from build123d import *

# Parameters (mm, degrees)
BOSS_EXTRUDE1_DEPTH      = 16.9
SKETCH2_W                = 6.8
SKETCH2_H                = 5
SKETCH2_R                = 1.7
BOSS_EXTRUDE2_DEPTH      = 2
BOSS_EXTRUDE2_2_DEPTH    = 2
BOSS_EXTRUDE3_REACH      = 37.726
BOSS_EXTRUDE3_END_RADIUS = 12.47
SKETCH5_W                = 2
SKETCH5_H                = 6.8
SKETCH7_W                = 6.8
SKETCH7_H                = 5
SKETCH7_R                = 1.7
BOSS_EXTRUDE4_DEPTH      = 2
BOSS_EXTRUDE4_2_DEPTH    = 2
BOSS_EXTRUDE5_REACH      = 37.726
BOSS_EXTRUDE5_END_RADIUS = 12.47
SKETCH8_W                = 2
SKETCH8_H                = 6.8
BOSS_EXTRUDE7_DEPTH      = 17
BOSS_EXTRUDE7_DEPTH_BACK = 23
SKETCH9_W                = 16.9
SKETCH9_H                = 2
CUT_EXTRUDE1_REACH       = 44.835
SKETCH10_R               = 1.7
FILLET1_R                = 2


with BuildPart() as part:
    # Sketch1 → Boss-Extrude1 (new body)
    with BuildSketch(Plane.XY):
        with BuildLine():
            ThreePointArc((9.47, 0), (-6.332886388, -7.040983596), (-1, 9.417053679))
            Line((-1, 9.417053679), (-1, 12.429839098))
            ThreePointArc((-1, 12.429839098), (-12.428769746, 1.01320413), (-3, -12.103755616))
            Line((-3, -12.103755616), (-3, -16.47))
            Line((-3, -16.47), (3, -16.47))
            Line((3, -16.47), (3, -12.103755616))
            ThreePointArc((3, -12.103755616), (12.428769746, 1.01320413), (1, 12.429839098))
            Line((1, 12.429839098), (1, 9.417053679))
            ThreePointArc((1, 9.417053679), (7.040983596, 6.332886388), (9.47, 0))
        make_face()
    extrude(amount=BOSS_EXTRUDE1_DEPTH)



with BuildPart() as body_2:
    # Sketch2 → Boss-Extrude2 (new body)
    with BuildSketch(Plane(origin=(-1, 0, 0), x_dir=(0, 0, -1), z_dir=(1, 0, 0))):
        with Locations((-13.5, 14.929839098)):
            Rectangle(SKETCH2_W, SKETCH2_H)
        with Locations((-13.5, 14.929839098)):
            Circle(SKETCH2_R, mode=Mode.SUBTRACT)
    extrude(amount=-BOSS_EXTRUDE2_DEPTH)


with BuildPart() as body_3:
    # Sketch2 → Boss-Extrude2 2 (new body)
    with BuildSketch(Plane(origin=(-1, 0, 0), x_dir=(0, 0, -1), z_dir=(1, 0, 0))):
        with Locations((-3.4, 14.929839098)):
            Rectangle(SKETCH2_W, SKETCH2_H)
        with Locations(Location((-3.4, 14.929839098, 0), (0, 0, 180))):
            Circle(SKETCH2_R, mode=Mode.SUBTRACT)
    extrude(amount=-BOSS_EXTRUDE2_2_DEPTH)


with BuildPart() as part_1:
    add(part.part)

    add(body_2.part)  # Boss-Extrude3 merges body 2

    add(body_3.part)  # Boss-Extrude3 merges body 3
    # Boss-Extrude3: up to this cylinder (the profile starts outside it)
    boss_extrude3_end = Plane(origin=(0, 0, 8.45), z_dir=(0, 0, -1)) * Cylinder(BOSS_EXTRUDE3_END_RADIUS, 111.492, mode=Mode.PRIVATE)
    # Sketch5 → Boss-Extrude3 (add, up to the surface)
    with BuildSketch(Plane.XZ.offset(-12.429839098), mode=Mode.PRIVATE) as boss_extrude3_sk1:
        with Locations((-2, 3.4)):
            Rectangle(SKETCH5_W, SKETCH5_H)
    boss_extrude3_tool1 = extrude(boss_extrude3_sk1.sketch, amount=BOSS_EXTRUDE3_REACH, mode=Mode.PRIVATE) - boss_extrude3_end
    add(boss_extrude3_tool1.solids().sort_by_distance((-2, 12.429839, 3.4))[0])
    # Sketch5 → Boss-Extrude3 (add, up to the surface)
    with BuildSketch(Plane.XZ.offset(-12.429839098), mode=Mode.PRIVATE) as boss_extrude3_sk2:
        with Locations((-2, 13.5)):
            Rectangle(SKETCH5_W, SKETCH5_H)
    boss_extrude3_tool2 = extrude(boss_extrude3_sk2.sketch, amount=BOSS_EXTRUDE3_REACH, mode=Mode.PRIVATE) - boss_extrude3_end
    add(boss_extrude3_tool2.solids().sort_by_distance((-2, 12.429839, 13.5))[0])



with BuildPart() as body_2_2:
    # Sketch7 → Boss-Extrude4 (new body)
    with BuildSketch(Plane.ZY.offset(-1)):
        with Locations((3.4, 14.929839098)):
            Rectangle(SKETCH7_W, SKETCH7_H)
        with Locations((3.4, 14.929839098)):
            Circle(SKETCH7_R, mode=Mode.SUBTRACT)
    extrude(amount=-BOSS_EXTRUDE4_DEPTH)


with BuildPart() as body_3_2:
    # Sketch7 → Boss-Extrude4 2 (new body)
    with BuildSketch(Plane.ZY.offset(-1)):
        with Locations((13.5, 14.929839098)):
            Rectangle(SKETCH7_W, SKETCH7_H)
        with Locations(Location((13.5, 14.929839098, 0), (0, 0, 180))):
            Circle(SKETCH7_R, mode=Mode.SUBTRACT)
    extrude(amount=-BOSS_EXTRUDE4_2_DEPTH)


with BuildPart() as part_2:
    add(part_1.part)

    add(body_2_2.part)  # Boss-Extrude5 merges body 2 2

    add(body_3_2.part)  # Boss-Extrude5 merges body 3 2
    # Boss-Extrude5: up to this cylinder (the profile starts outside it)
    boss_extrude5_end = Plane(origin=(0, 0, 8.45), z_dir=(0, 0, -1)) * Cylinder(BOSS_EXTRUDE5_END_RADIUS, 111.492, mode=Mode.PRIVATE)
    # Sketch8 → Boss-Extrude5 (add, up to the surface)
    with BuildSketch(Plane.XZ.offset(-12.429839098), mode=Mode.PRIVATE) as boss_extrude5_sk1:
        with Locations((2, 3.4)):
            Rectangle(SKETCH8_W, SKETCH8_H)
    boss_extrude5_tool1 = extrude(boss_extrude5_sk1.sketch, amount=BOSS_EXTRUDE5_REACH, mode=Mode.PRIVATE) - boss_extrude5_end
    add(boss_extrude5_tool1.solids().sort_by_distance((2, 12.429839, 3.4))[0])
    # Sketch8 → Boss-Extrude5 (add, up to the surface)
    with BuildSketch(Plane.XZ.offset(-12.429839098), mode=Mode.PRIVATE) as boss_extrude5_sk2:
        with Locations((2, 13.5)):
            Rectangle(SKETCH8_W, SKETCH8_H)
    boss_extrude5_tool2 = extrude(boss_extrude5_sk2.sketch, amount=BOSS_EXTRUDE5_REACH, mode=Mode.PRIVATE) - boss_extrude5_end
    add(boss_extrude5_tool2.solids().sort_by_distance((2, 12.429839, 13.5))[0])

    # Sketch9 → Boss-Extrude7 (add, two sides: drawn at the far end of the back side and taken through both)
    with BuildSketch(Plane.ZY.offset(3).offset(-BOSS_EXTRUDE7_DEPTH_BACK)):
        with Locations((8.45, -15.47)):
            Rectangle(SKETCH9_W, SKETCH9_H)
    extrude(amount=BOSS_EXTRUDE7_DEPTH + BOSS_EXTRUDE7_DEPTH_BACK)

    # Sketch10 → Cut-Extrude1 (cut, up to next)
    with BuildSketch(Plane.XZ.offset(16.47), mode=Mode.PRIVATE) as cut_extrude1_sk1:
        with Locations(Location((-15, 3.45, 0), (0, 0, 270))):
            Circle(SKETCH10_R)
    cut_extrude1_tool1 = extrude(cut_extrude1_sk1.sketch, amount=-CUT_EXTRUDE1_REACH, mode=Mode.PRIVATE) & part_2.part
    # Sketch10 → Cut-Extrude1 (cut, up to next)
    with BuildSketch(Plane.XZ.offset(16.47), mode=Mode.PRIVATE) as cut_extrude1_sk2:
        with Locations(Location((-15, 13.45, 0), (0, 0, 270))):
            Circle(SKETCH10_R)
    cut_extrude1_tool2 = extrude(cut_extrude1_sk2.sketch, amount=-CUT_EXTRUDE1_REACH, mode=Mode.PRIVATE) & part_2.part
    # Sketch10 → Cut-Extrude1 (cut, up to next)
    with BuildSketch(Plane.XZ.offset(16.47), mode=Mode.PRIVATE) as cut_extrude1_sk3:
        with Locations(Location((15, 3.45, 0), (0, 0, 270))):
            Circle(SKETCH10_R)
    cut_extrude1_tool3 = extrude(cut_extrude1_sk3.sketch, amount=-CUT_EXTRUDE1_REACH, mode=Mode.PRIVATE) & part_2.part
    # Sketch10 → Cut-Extrude1 (cut, up to next)
    with BuildSketch(Plane.XZ.offset(16.47), mode=Mode.PRIVATE) as cut_extrude1_sk4:
        with Locations(Location((15, 13.45, 0), (0, 0, 270))):
            Circle(SKETCH10_R)
    cut_extrude1_tool4 = extrude(cut_extrude1_sk4.sketch, amount=-CUT_EXTRUDE1_REACH, mode=Mode.PRIVATE) & part_2.part
    add(cut_extrude1_tool1.solids().sort_by_distance((-15, -16.47, 3.45))[0], mode=Mode.SUBTRACT)
    add(cut_extrude1_tool2.solids().sort_by_distance((-15, -16.47, 13.45))[0], mode=Mode.SUBTRACT)
    add(cut_extrude1_tool3.solids().sort_by_distance((15, -16.47, 3.45))[0], mode=Mode.SUBTRACT)
    add(cut_extrude1_tool4.solids().sort_by_distance((15, -16.47, 13.45))[0], mode=Mode.SUBTRACT)

    # Fillet1
    # the kernel refuses this fillet: 2 mm, written as the material it adds along each edge
    with BuildSketch(Plane(origin=(-3, -12.103755616, 0), x_dir=(-0.9559582766785055, 0.2935025949627393, 0), z_dir=(0, 0, 1))) as fillet1_piece_1:
        with BuildLine():
            CenterArc((1.479018642, 1.996983664), FILLET1_R, 197.067768115, 69.785084401)
            Line((-0.432897911, 1.409978474), (0, 0))
            ThreePointArc((0, 0), (0.684608852, 0.018806856), (1.369217704, 0))
        make_face()
    extrude(amount=16.9)
    with BuildSketch(Plane(origin=(-3, -14.47, 16.9), x_dir=(0, 1, 0), z_dir=(0, 0, -1))) as fillet1_piece_2:
        with BuildLine():
            CenterArc((FILLET1_R, -FILLET1_R), FILLET1_R, 90, 90)
            Line((0, -FILLET1_R), (0, 0))
            Line((0, 0), (FILLET1_R, 0))
        make_face()
    extrude(amount=16.9)
    with BuildSketch(Plane(origin=(3, -12.103755616, 0), x_dir=(0.9559582766785055, 0.2935025949627393, 0), z_dir=(0, 0, 1))) as fillet1_piece_3:
        with BuildLine():
            CenterArc((1.479018642, -1.996983664), FILLET1_R, 93.147147485, 69.785084401)
            Line((-0.432897911, -1.409978474), (0, 0))
            ThreePointArc((0, 0), (0.684608852, -0.018806856), (1.369217704, 0))
        make_face()
    extrude(amount=16.9)
    with BuildSketch(Plane(origin=(3, -14.47, 0), x_dir=(1, 0, 0), z_dir=(0, 0, 1))) as fillet1_piece_4:
        with BuildLine():
            CenterArc((FILLET1_R, FILLET1_R), FILLET1_R, 180, 90)
            Line((0, FILLET1_R), (0, 0))
            Line((0, 0), (FILLET1_R, 0))
        make_face()
    extrude(amount=16.9)


solid = part_2.part
CAD build for the part. Positions are in the model's coordinates, mm. A direction names the side the tool comes from. Round coordinates to 2 decimals unless told otherwise and drop trailing zeros. Order: outer loops, then holes, each group sorted by start corner. A loop starts at its lowest first (then second) coordinate and runs counter-clockwise, first axis right, second up. Notation, with made-up numbers: (57, 0.5) -> (65, 0.5) arc R21 ccw to (65, 4.5) -> close; hole circle Ø1 at (58, 87). An arc over 180 degrees is marked (long way). Write each question's results on one line, items separated by ' | '.
1. Cut at B-B (x = 15). Give the cut face in (y, z).
Findings below:
outline: (-16.47, 0) -> (-14.47, 0) -> (-14.47, 1.75) -> (-16.47, 1.75) -> close; (-16.47, 5.15) -> (-14.47, 5.15) -> (-14.47, 11.75) -> (-16.47, 11.75) -> close; (-16.47, 15.15) -> (-14.47, 15.15) -> (-14.47, 16.9) -> (-16.47, 16.9) -> close
2. Cut at C-C (y = -2). Give the cut face in (x, z).
Findings below:
outline: (-12.31, 0) -> (-9.26, 0) -> (-9.26, 16.9) -> (-12.31, 16.9) -> close; (9.26, 0) -> (12.31, 0) -> (12.31, 16.9) -> (9.26, 16.9) -> close
3. 3-axis set-ups, long thin cutter, end or side, ignore diameter. For faces 1 (the face through (-3, 13, 13)), 2 (the face through (3, 13, 13)), 3 (the face through (-3.527, -12.226, 8.332)): which of +Z, -Z, +X, -X, +Y, -Y reach the whole face in a straight line?
Findings below:
face 1: +Z, -Z, -X, +Y | face 2: +Z, -Z, +X, +Y | face 3: +Z, -Z, -X
4. Cut at D-D (z = 14.25). Count the separate pieces of the cut face and the enclosed holes in it, plus the area to 3 significant figures.
Findings below:
separate pieces: 5 | enclosed holes: 0 | area: 292 mm²
5. Flat gauge pins, fed straight in: P1, Ø5, axis at x = 2.5, y = 6, coming from the -Z side; P2, Ø4.5, axis at x = -15.5, z = 11.5, coming from the +Y side; P3, Ø5, axis at x = 8.5, z = 14.5, coming from the +Y side; P4, Ø9, axis at y = 12.5, z = 5.5, coming from the -X side. Where does each tip first touch, or does it go through?
Findings below:
P1: passes through | P2: stops at y = -14.47 | P3: stops at y = 10.93 | P4: stops at x = -9.57
6. Pull direction Y, two halves, no side cores. Call faces 4 (the face through (0, -16.47, 8)), 5 (the face through (-3, 13, 3)), 6 (the face through (-1.99, 15.96, 2.05)): pulls with the +Y half, pulls with the -Y half, needs draft (parallel to the pull), parting line crosses it, or undercut.
Findings below:
face 4: pulls with the -Y half | face 5: needs draft | face 6: undercut
7. Cut at A-A (x = 2). Give the cut face in (y, z), plus the area to 3 significant figures.
Findings below:
outline: (-16.47, 0) -> (-9.26, 0) -> (-9.26, 16.9) -> (-16.47, 16.9) -> close; (9.26, 0) -> (17.43, 0) -> (17.43, 6.8) -> (12.31, 6.8) -> (12.31, 10.1) -> (17.43, 10.1) -> (17.43, 16.9) -> (9.26, 16.9) -> close; hole circle Ø3.4 at (14.93, 3.4); hole circle Ø3.4 at (14.93, 13.5) | area: 225 mm²
8. Wall check: line 1 along X through (y, z) = (-15.7, 3.45); line 2 along Y through (x, z) = (-2.5, 14.25); line 3 along Y through (x, z) = (-8, 1). Give the ranges that are in metal, low to high. Write a range as [from, to].
Findings below:
line 1: x = [-20, -16.7], [-13.3, 13.3], [16.7, 20] | line 2: y = [-16.47, -9.13], [9.13, 13.4], [16.46, 17.43] | line 3: y = [-16.47, -14.47], [-9.57, -5.07], [5.07, 9.57]
